from build123d import *

# Parameters (mm, degrees)
EXTRUDE_1_DEPTH = 4


with BuildPart() as part:
    # Sketch 1 → Бобышка-Вытянуть1 (new body)
    with BuildSketch(Plane(origin=(26.561401347, 0, 21.984207178), x_dir=(-0.9674249636260779, -8.775997465141552e-15, 0.25315793440672957), z_dir=(0, 1, 0))):
        Polygon((0, 0), (7.088422163, 27.087898982), (110.602893271, 0), (103.514471108, -27.087898982), align=None)
        Polygon((9.855076732, 13.959851812), (6.310865651, 0.415902321), (19.854815141, -3.128308761), (23.399026223, 10.41564073), align=None, mode=Mode.SUBTRACT)
        Polygon((105.630148131, -11.102783695), (102.08593705, -24.646733185), (88.541987559, -21.102522104), (92.08619864, -7.558572613), align=None, mode=Mode.SUBTRACT)
        Polygon((89.18392375, -6.79909881), (85.639712668, -20.343048301), (72.095763177, -16.798837219), (75.639974259, -3.254887728), align=None, mode=Mode.SUBTRACT)
        Polygon((69.193488286, -16.039363416), (55.649538795, -12.495152334), (59.193749877, 1.048797157), (72.737699368, -2.495413925), align=None, mode=Mode.SUBTRACT)
        Polygon((52.747263905, -11.735678531), (56.291474986, 1.80827096), (42.747525496, 5.352482042), (39.203314414, -8.191467449), align=None, mode=Mode.SUBTRACT)
        Polygon((39.845250605, 6.111955845), (26.301301114, 9.656166927), (22.757090032, -3.887782564), (36.301039523, -7.431993646), align=None, mode=Mode.SUBTRACT)
    extrude(amount=EXTRUDE_1_DEPTH)


solid = part.part
Build history of the part. All positions in model axes, mm. A direction names the side the tool comes from. Round coordinates to 2 decimals unless told otherwise and drop trailing zeros. Write each loop counter-clockwise with the first axis right and the second up, starting at its lowest first coordinate (ties: lowest second). Pieces come first, ordered by that corner, then holes. Notation, with made-up numbers: M -7.5,7.5 L 45.5,7.5 A16 ccw 45.5,26.5 Z; hole C -32.75,18 d2. An arc over 180 degrees is marked long. Answer as a JSON object with one key per item and string values. Group by question number.
(1) Cut at B-B (x = -8.5). Give the cut face in (y, z), and give its area (3 significant figures).
(2) Drill centre line: L1, parallel to Z at x = -60, y = 1.3. Where is it in solid material? Low to high.
(3) Mould opens along X. For faces 1 (the flat face through (-26, 2, 49.984)), 2 (the flat face through (26.561, 2, 36)), 3 (the flat face through (-72, 2, 23.984)) say: pulls with the +X half, pulls with the -X half, needs draft (parallel to the pull), parting line crosses it, or undercut.
(4) Cut at C-C (y = 1.55). Give the cut face in (x, z).
(5) Cut at A-A (z = 33). Give the cut face in (x, y).
(6) Which spindle directions (+Z, -Z, +X, -X, +Y, -Y) get a long thin tool onto all of the face, cutting with end or side? Do faces 4 (the flat face through (-21, 2, 37.984)), 5 (the flat face through (-26, 4, 42)). Say none if no direction does.
Responses:
{
 "1": {"outline": "M 0,21.98 L 4,21.98 L 4,23.98 L 0,23.98 Z; M 0,37.98 L 4,37.98 L 4,49.98 L 0,49.98 Z", "area": "56.0 mm2"},
 "2": {"L1": "z = 21.98 to 23.98, 37.98 to 49.98"},
 "3": {"face 1": "needs draft", "face 2": "pulls with the +X half", "face 3": "undercut"},
 "4": {"outline": "M -80.44,21.98 L 26.56,21.98 L 26.56,49.98 L -80.44,49.98 Z; hole M -78.44,23.98 L -64.44,23.98 L -64.44,37.98 L -78.44,37.98 Z; hole M -61.44,23.98 L -47.44,23.98 L -47.44,37.98 L -61.44,37.98 Z; hole M -44.44,23.98 L -30.44,23.98 L -30.44,37.98 L -44.44,37.98 Z; hole M -27.44,23.98 L -13.44,23.98 L -13.44,37.98 L -27.44,37.98 Z; hole M -10.44,23.98 L 3.56,23.98 L 3.56,37.98 L -10.44,37.98 Z; hole M 6.56,23.98 L 20.56,23.98 L 20.56,37.98 L 6.56,37.98 Z"},
 "5": {"outline": "M -80.44,0 L -78.44,0 L -78.44,4 L -80.44,4 Z; M -64.44,0 L -61.44,0 L -61.44,4 L -64.44,4 Z; M -47.44,0 L -44.44,0 L -44.44,4 L -47.44,4 Z; M -30.44,0 L -27.44,0 L -27.44,4 L -30.44,4 Z; M -13.44,0 L -10.44,0 L -10.44,4 L -13.44,4 Z; M 3.56,0 L 6.56,0 L 6.56,4 L 3.56,4 Z; M 20.56,0 L 26.56,0 L 26.56,4 L 20.56,4 Z"},
 "6": {"face 4": "+Y, -Y", "face 5": "+Z, -Z, +X, -X, +Y"}
}
